from build123d import *

# Parameters (mm, degrees)
SKETCH1_W           = 50
SKETCH1_H           = 23
BOSS_EXTRUDE1_DEPTH = 20
SKETCH2_W           = 17
SKETCH2_H           = 17
CUT_EXTRUDE1_DEPTH  = 56.065869647
BOSS_EXTRUDE2_DEPTH = 3
SKETCH4_R           = 1.75
SKETCH4_R_2         = 3.5
SKETCH4_R_3         = 2
CUT_EXTRUDE4_DEPTH  = 57.484511151
FILLET1_R           = 20


with BuildPart() as part:
    # Sketch1 → Boss-Extrude1 (new body)
    with BuildSketch(Plane(origin=(0, 0, 0), x_dir=(1, 0, 0), z_dir=(0, 1, 0))):
        Rectangle(SKETCH1_W, SKETCH1_H)
    extrude(amount=BOSS_EXTRUDE1_DEPTH)

    # Sketch2 → Cut-Extrude1 (cut, through all)
    with BuildSketch(Plane(origin=(25, 0, 0), x_dir=(0, 0, -1), z_dir=(1, 0, 0))):
        with Locations((0, 8.5)):
            Rectangle(SKETCH2_W, SKETCH2_H)
    extrude(amount=-CUT_EXTRUDE1_DEPTH, mode=Mode.SUBTRACT)

    # Sketch3 → Boss-Extrude2 (add)
    with BuildSketch(Plane(origin=(0, 20, 0), x_dir=(1, 0, 0), z_dir=(0, 1, 0))):
        with BuildLine():
            Line((25, 15.5), (35, 15.5))
            ThreePointArc((35, 15.5), (50.5, 0), (35, -15.5))
            Line((35, -15.5), (25, -15.5))
            Line((25, -15.5), (10, -11.5))
            Line((10, -11.5), (25, -11.5))
            Line((25, -11.5), (25, 11.5))
            Line((25, 11.5), (10, 11.5))
            Line((10, 11.5), (25, 15.5))
        make_face()
    extrude(amount=-BOSS_EXTRUDE2_DEPTH)

    # Sketch4 → Cut-Extrude4 (cut, through all)
    with BuildSketch(Plane(origin=(0, 20, 0), x_dir=(1, 0, 0), z_dir=(0, 1, 0))):
        with Locations(Location((-15, 0, 0), (0, 0, 270))):
            Circle(SKETCH4_R)
        with Locations(Location((-5, 0, 0), (0, 0, 270))):
            Circle(SKETCH4_R)
        with Locations(Location((35, 0, 0), (0, 0, 270))):
            Circle(SKETCH4_R_2)
        with Locations(Location((28.282485579, -6.717514421, 0), (0, 0, 270))):
            Circle(SKETCH4_R_3)
        with Locations(Location((41.717514421, 6.717514421, 0), (0, 0, 270))):
            Circle(SKETCH4_R_3)
        with Locations(Location((40.727564928, -5.727564928, 0), (0, 0, 270))):
            Circle(SKETCH4_R_3)
        with Locations(Location((29.272435072, 5.727564928, 0), (0, 0, 270))):
            Circle(SKETCH4_R_3)
    extrude(amount=-CUT_EXTRUDE4_DEPTH, mode=Mode.SUBTRACT)

    # Fillet1
    fillet1_edges = [part.edges().sort_by_distance(p)[0] for p in [
        (25, 18.5, -15.5),
        (25, 18.5, 15.5),
    ]]
    fillet(fillet1_edges, radius=FILLET1_R)


solid = part.part
Read the model definition and answer for the solid it produces. Units are mm, in the model's axes. A direction names the side the tool comes from. Round coordinates to 2 decimals unless told otherwise and drop trailing zeros. Write each loop counter-clockwise with the first axis right and the second up, starting at its lowest first coordinate (ties: lowest second). Pieces come first, ordered by that corner, then holes. Notation, with made-up numbers: (0, 41) - (41, 41) arc R19 cw to (41, 78) - close; hole circle Ø11 at (61, 36.25). An arc over 180 degrees is marked (long way). One line per question, with ' | ' between items. Start each with the question number.
1. Section B-B (y = 16.25) is taken. Determine the outline of the cut face in (x, z), and give its area (3 significant figures).
2. Each of these flat-tipped pins is pushed along its axis until it touches: pin 1 (8 mm diameter, centred on y = 11.5, z = -8, fed in from +X); pin 2 (8.5 mm diameter, centred on x = 7, y = 9, fed in from -Z); pin 3 (5 mm diameter, centred on x = 36.5, z = 11, fed in from -Y); pin 4 (15.5 mm diameter, centred on x = 24, z = -2.5, fed in from -Y). Where does it stop, or does it pass through?
3. Section A-A (x = -15) is taken. Determine the outline of the cut face in (y, z), and give its area (4 significant figures).
4. Section D-D (z = -5.5) is taken. Determine the outline of the cut face in (x, y).
5. Find the intervals of material crossed by probe 1 along X at (y, z) = (19.3, 0); probe 2 along Z at (x, y) = (-5.5, 8); probe 3 along X at (y, z) = (11, -10), in increasing order. Write a range as [from, to].
6. Section C-C (z = 0) is taken. Determine the outline of the cut face in (x, y).
7. For faces 5 (the face through (25, 8, -10)), 6 (the face through (13, 20, 0)), determine the directions among +Z, -Z, +X, -X, +Y, -Y from which every point of the face is accessible in a straight line to the end or side of a thin tool.
8. For a pull along Z with two mould halves and no side action, classify faces 1 (the face through (27.32, 18.52, -6.16)), 2 (the face through (0, 0, 10)), 3 (the face through (16.321, 18.521, 13.186)), 4 (the face through (30.265, 18.521, 6.457)) as +Z half, -Z half, draft (parallel to the pull), parting line (faces both ways), or undercut.
Filled in:
1) outline: (-25, -11.5) - (25, -11.5) - (25, -8.5) - (-25, -8.5) - close; (-25, 8.5) - (25, 8.5) - (25, 11.5) - (-25, 11.5) - close | area: 300 mm²
2) pin 1: x = 25 | pin 2: z = -11.5 | pin 3: y = 17 | pin 4: y = 0
3) outline: (0, -11.5) - (20, -11.5) - (20, -1.75) - (17, -1.75) - (17, -8.5) - (0, -8.5) - close; (0, 8.5) - (17, 8.5) - (17, 1.75) - (20, 1.75) - (20, 11.5) - (0, 11.5) - close | area: 160.5 mm²
4) outline: (-25, 17) - (27.29, 17) - (27.29, 20) - (-25, 20) - close; (31.26, 17) - (40.13, 17) - (40.13, 20) - (31.26, 20) - close; (43.3, 17) - (49.49, 17) - (49.49, 20) - (43.3, 20) - close
5) probe 1: [-25, -16.75], [-13.25, -6.75], [-3.25, 31.5], [38.5, 50.5] | probe 2: [-11.5, -8.5], [8.5, 11.5] | probe 3: [-25, 25]
6) outline: (-25, 17) - (-16.75, 17) - (-16.75, 20) - (-25, 20) - close; (-13.25, 17) - (-6.75, 17) - (-6.75, 20) - (-13.25, 20) - close; (-3.25, 17) - (31.5, 17) - (31.5, 20) - (-3.25, 20) - close; (38.5, 17) - (50.5, 17) - (50.5, 20) - (38.5, 20) - close
7) face 5: +Z, -Z, +X, -Y | face 6: +Z, -Z, +X, -X, +Y
8) face 1: undercut | face 2: draft | face 3: +Z half | face 4: undercut
